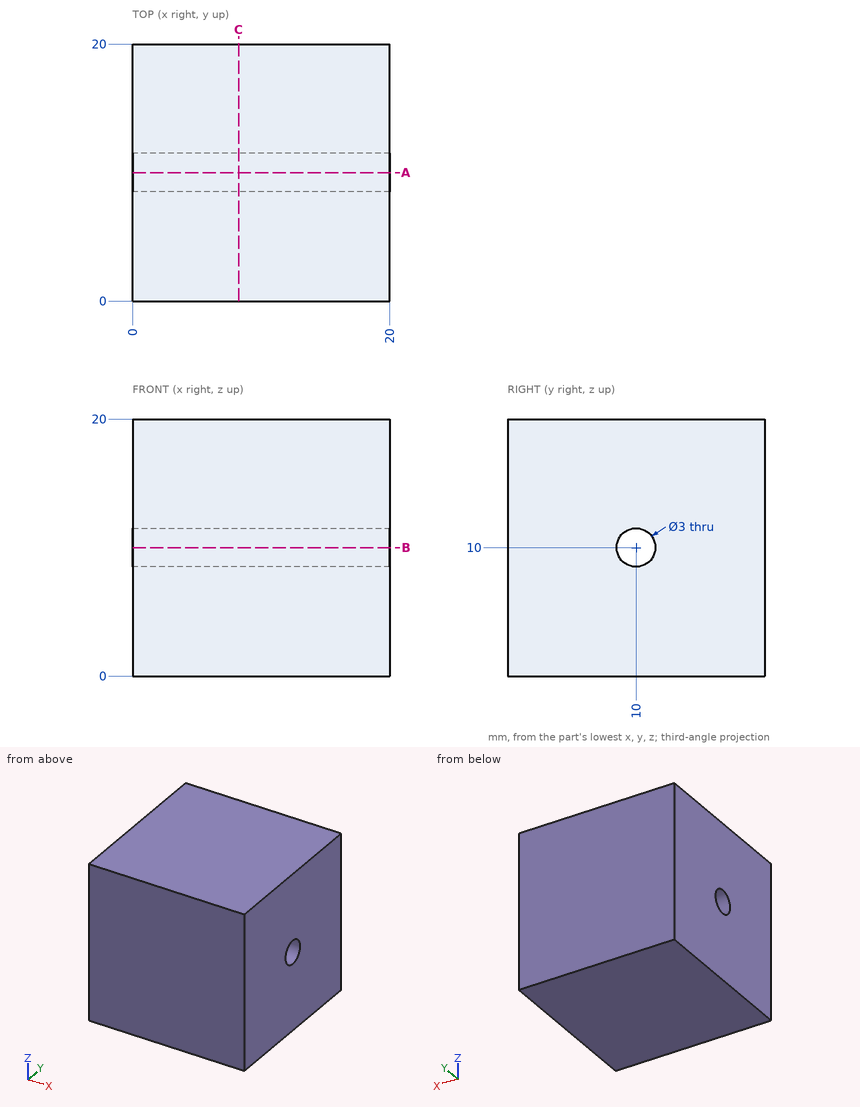
Could you check a few things on this drawing? It's one solid part, dimensions in mm from its lowest x, y, z. Round coordinates to 2 decimals unless told otherwise and drop trailing zeros. Order: outer loops, then holes, each group sorted by start corner. A loop starts at its lowest first (then second) coordinate and runs counter-clockwise, first axis right, second up.
(1) Imagine slicing it at A-A (y = 10). Write out the boundary of the cut face in (x, z), plus the area to 3 significant figures.
Response values:
outline: (0, 0) - (20, 0) - (20, 8.5) - (0, 8.5) - close; (0, 11.5) - (20, 11.5) - (20, 20) - (0, 20) - close
area: 340 mm2
(2) Please list where this line runs through material, in increasing order: line 1 along Y through (x, z) = (8.75, 10).
Response values:
line 1: y = 0 to 8.5, 11.5 to 20
(3) I'm going to push flat-ended pins straight in: pin 1 (8 mm diameter, centred on y = 18, z = 10, fed in from -X); pin 2 (2.5 mm diameter, centred on y = 10, z = 10, fed in from +X). Where does each tip first touch, or does it pass through?
Response values:
pin 1: stops at x = 0
pin 2: passes through
(4) Imagine slicing it at C-C (x = 8.25). Write out the boundary of the cut face in (y, z).
Response values:
outline: (0, 0) - (20, 0) - (20, 20) - (0, 20) - close; hole circle Ø3 at (10, 10)
